The model under review builds one solid part; all positions refer to its coordinate system, in mm. Face numbers are marked on the shaded views. A direction names the side the tool comes from. Give positions to 0.01 mm unless a question says otherwise; leave off trailing zeros. Loops run counter-clockwise (first coordinate to the right, second up) from the corner with the lowest first, then second, coordinate; pieces in that order, holes last. Notation, with made-up numbers: (-12, -10) - (4, -10) arc R19 ccw to (4, 10) - close; hole circle Ø10 at (-25.75, -30.75). An arc over 180 degrees is marked (long way). Answer as a JSON object with one key per item and string values.
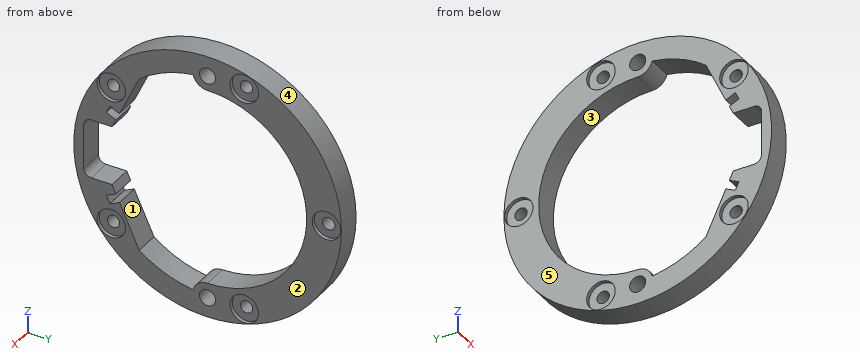
Autodesk Inventor part; units mm, degrees
ref_plane "YZ Plane" through (0, 0, 0) normal (1, 0, 0) x (0, 1, 0)
ref_plane "XZ Plane" through (0, 0, 0) normal (0, 1, 0) x (-1, 0, 0)
ref_plane "XY Plane" through (0, 0, 0) normal (0, 0, 1) x (1, 0, 0)
sketch "Sketch1" plane through (0, 0, 0) normal (1, 0, 0) x (0, 1, 0)
  circle A0 centre (-0.0138, -0.0327) radius 54
  circle A1 centre (-0.0138, 45.9673) radius 3.25
  circle A2 centre (-0.0138, -46.0327) radius 3.25
  arc A3 (-5.855, 44.5961) -> (-0.0138, 39.9673) centre (-0.0138, 45.9673) ccw
  arc A4 (-0.0138, -40.0327) -> (-5.8512, -44.6455) centre (-0.0138, -46.0327) ccw
  arc A5 (-0.0138, -40.0327) -> (-0.0138, 39.9673) centre (-0.0138, -0.0327) ccw
  line L0 (-38.5532, 11.9673) -> (-49.9975, 11.9673)
  line L1 (-49.9975, 11.9673) -> (-49.9975, -12.0327)
  line L2 (-38.5532, -12.0327) -> (-49.9975, -12.0327)
  arc A6 (-5.855, 44.5961) -> (-27.5449, 35.5747) centre (-0.0138, -0.0327) ccw
  arc A7 (-27.56, -35.6078) -> (-5.8512, -44.6455) centre (-0.0138, -0.0327) ccw
  line L3 (-36.9846, 15.3313) -> (-40.8817, 17.1485)
  line L4 (-40.8817, 17.1485) -> (-39.4448, 20.23)
  line L5 (-39.4448, 20.23) -> (-35.5477, 18.4127)
  line L6 (-35.5477, 18.4127) -> (-27.5449, 35.5747)
  line L7 (-36.9846, 15.3313) -> (-38.5532, 11.9673)
  line L8 (-36.9846, -15.3967) -> (-40.8817, -17.214)
  line L9 (-40.8817, -17.214) -> (-39.4448, -20.2954)
  line L10 (-39.4448, -20.2954) -> (-35.5477, -18.4782)
  line L11 (-36.9846, -15.3967) -> (-38.5532, -12.0327)
  line L12 (-35.5477, -18.4782) -> (-27.56, -35.6078)
  line L13 (-0.0138, -0.0327) -> (-40.1632, 18.6893)
  line L14 (-0.0138, -0.0327) -> (-40.1632, -18.7547)
  line L15 (-0.0138, -0.0327) -> (-50.798, -0.0327) construction
  line L16 (-0.0138, -0.0327) -> (50.7703, -0.0327) construction
  dimension "d4" = 6.5
  dimension "d5" = 6.5
  dimension "d25" = 24
  dimension "d27" = 4.3
  dimension "d28" = 3.4
  dimension "d31" = 4.3
  dimension "d32" = 3.4
  dimension "d39" = 90
  dimension "d40" = 90
  dimension "d41" = 90
  dimension "d42" = 90
  dimension "d44" = 90
  dimension "d45" = 90
  dimension "d67" = 40
  dimension "d68" = 40
  dimension "d70" = 4.3
  dimension "d71" = 1.7
  dimension "d72" = 4.3
  dimension "d73" = 90
  dimension "d74" = 90
  dimension "d76" = 108
  dimension "d81" = 40
  dimension "d93" = 46
  dimension "d94" = 46
  dimension "d95" = 6
  dimension "d96" = 6
  dimension "d97" = 180
  dimension "d98" = 12
  dimension "d99" = 12
  dimension "d100" = 25
  dimension "d101" = 25
  dimension "d102" = 1.7
extrude "Extrusion1" add sketch "Sketch1" along normal blind 10
fillet "Fillet1" radius 3 2 edges at (5, -49.9975, 11.9673) (5, -49.9975, -12.0327)
sketch "Sketch2" plane through (10, -0.0138, -0.0327) normal (1, 0, 0) x (0, 0, -1)
  circle A0 centre (0, 0) radius 48
  circle A1 centre (0, 48) radius 2.5
  arc A2 (40, 0) -> (-40, 0) centre (0, 0) ccw
  arc A3 (40, 0) -> (44.6128, -5.8374) centre (46, 0) ccw
  arc A4 (35.575, -27.5462) -> (44.6128, -5.8374) centre (0, 0) ccw
  line L0 (35.575, -27.5462) -> (18.4455, -35.5339)
  line L1 (18.4455, -35.5339) -> (20.2627, -39.431)
  line L2 (20.2627, -39.431) -> (17.1813, -40.8679)
  line L3 (17.1813, -40.8679) -> (15.364, -36.9708)
  line L4 (15.364, -36.9708) -> (12, -38.5394)
  line L5 (12, -38.5394) -> (12, -46.9837)
  arc A5 (9, -49.9837) -> (12, -46.9837) centre (9, -46.9837) ccw
  line L6 (9, -49.9837) -> (-9, -49.9837)
  arc A6 (-12, -46.9837) -> (-9, -49.9837) centre (-9, -46.9837) ccw
  line L7 (-12, -46.9837) -> (-12, -38.5394)
  line L8 (-12, -38.5394) -> (-15.364, -36.9708)
  line L9 (-15.364, -36.9708) -> (-17.1813, -40.8679)
  line L10 (-17.1813, -40.8679) -> (-20.2627, -39.431)
  line L11 (-20.2627, -39.431) -> (-18.4455, -35.5339)
  line L12 (-18.4455, -35.5339) -> (-35.6074, -27.5311)
  arc A7 (-44.6288, -5.8412) -> (-35.6074, -27.5311) centre (0, 0) ccw
  arc A8 (-44.6288, -5.8412) -> (-40, 0) centre (-46, 0) ccw
  circle A9 centre (46, 0) radius 3.25
  circle A10 centre (-46, 0) radius 3.25
  circle A11 centre (0, 0) radius 54
  circle A12 centre (0, 0) radius 54
  circle A13 centre (-45.6507, 14.8328) radius 2.5
  circle A14 centre (-28.2137, -38.8328) radius 2.5
  circle A15 centre (28.2137, -38.8328) radius 2.5
  circle A16 centre (45.6507, 14.8328) radius 2.5
  point P0 (-0.0327, 0.0138)
  dimension "d50" = 96
  dimension "d51" = 5
  dimension "d80" = 108
  dimension "d84" = 360
  dimension "d103" = 0
extrude "Extrusion2" cut sketch "Sketch2" against normal blind 10 contours A16 A0 | A0 A16 | A15 A0 | A0 A15 | A1 A0 | A0 A1 | A13 A0 | A0 A13 | A14 A0 | A0 A14
sketch "Sketch3" plane through (10, -0.0138, -0.0327) normal (1, 0, 0) x (0, 0, -1)
  circle A0 centre (0, 48) radius 2.5
  circle A1 centre (0, 48) radius 5.75
  circle A2 centre (0, 0) radius 54
  circle A3 centre (-45.6507, 14.8328) radius 5.75
  circle A4 centre (-28.2137, -38.8328) radius 5.75
  circle A5 centre (28.2137, -38.8328) radius 5.75
  circle A6 centre (45.6507, 14.8328) radius 5.75
  point P0 (-0.0327, 0.0138)
  dimension "d58" = 11.5
  dimension "d88" = 360
extrude "Extrusion3" cut sketch "Sketch3" against normal blind 1.5 contours A1 | A3 | A4 | A5 | A6
sketch "Sketch6" plane through (0, -0.0138, -0.0327) normal (-1, 0, 0) x (0, 0, 1)
  circle A0 centre (0, 48) radius 5.75
  circle A1 centre (-45.6507, 14.8328) radius 5.75
  circle A2 centre (-28.2137, -38.8328) radius 5.75
  circle A3 centre (28.2137, -38.8328) radius 5.75
  circle A4 centre (45.6507, 14.8328) radius 5.75
  point P0 (0.0327, 0.0138)
extrude "Extrusion5" cut sketch "Sketch6" against normal blind 1.5
equation "\"d98\" = 0.5 * d25"
properties part number "3219_Center Rung_V1" material "Acetal Resin, White"
Q1. Consider section A-A, the plane z = 29. State the section outline as (x, y) points, plus the area to 3 significant figures.
Results:
{"outline": "(0, -45.55) - (10, -45.55) - (10, -44.54) - (8.5, -44.54) - (8.5, -41.21) - (1.5, -41.21) - (1.5, -44.54) - (0, -44.54) - close; (0, -33.16) - (1.5, -33.16) - (1.5, -36.48) - (8.5, -36.48) - (8.5, -33.16) - (10, -33.16) - (10, -30.61) - (0, -30.61) - close; (0, 27.5) - (10, 27.5) - (10, 45.52) - (0, 45.52) - close", "area": "262 mm^2"}
Q2. Clearance check with flat-ended pins moving along their axes: pin 1 Ø6 at (y, z) = (13, -44) entering from +X; pin 2 Ø5 at (x, z) = (5.5, 33) entering from +Y; pin 3 Ø5 at (x, y) = (3, -9) entering from +Z. State where each tip first meets the part, or that it passes through.
Results:
{"pin 1": "stops at x = 8.5", "pin 2": "stops at y = 44.53", "pin 3": "stops at z = 53.58"}
Q3. Consider section C-C, the plane x = 5. State how many separate pieces and enclosed holes the cut face has, plus the area to 3 significant figures.
Results:
{"separate pieces": "1", "enclosed holes": "8", "area": "3,390 mm^2"}
Q4. For the marked faces 1 and 2, list the 3-axis set-ups (+Z, -Z, +X, -X, +Y, -Y) from which the entire face can be reached by the end or side of a thin tool; tool diameter is ignored.
Results:
{"face 1": "+X, -X", "face 2": "+Z, -Z, +X, +Y, -Y"}
Q5. The part is to be moulded in two halves that separate along Z. For the marked faces 3, 4 and 5, say which applies: +Z half, -Z half, draft (parallel to the pull), parting line (faces both ways), or undercut.
Results:
{"face 3": "undercut", "face 4": "parting line", "face 5": "draft"}
Q6. To check wall thickness, follow probe 1 along Y at (x, z) = (8.25, 1); probe 2 along Y at (x, z) = (3.75, 29); probe 3 along Z at (x, y) = (9, -12). State the ranges of each line that lie inside material, in increasing order. Write a range as [from, to].
Results:
{"probe 1": "y = [-54, -50], [39.97, 45.71], [50.26, 53.98]", "probe 2": "y = [-45.55, -41.21], [-36.48, -30.61], [27.5, 45.52]", "probe 3": "z = [-52.69, -43.4], [43.35, 52.62]"}
Q7. Consider section B-B, the plane y = 35.5. State the section outline as (x, z) points.
Results:
{"outline": "(0, -40.71) - (10, -40.71) - (10, -18.44) - (0, -18.44) - close; (0, 18.37) - (10, 18.37) - (10, 40.65) - (0, 40.65) - close"}
Q8. Consider section D-D, the plane y = -14.5. State the section outline as (x, z) points, plus the area to 3 significant figures.
Results:
{"outline": "(0, -52.05) - (10, -52.05) - (10, -42.63) - (0, -42.63) - close; (0, 42.58) - (10, 42.58) - (10, 51.99) - (0, 51.99) - close", "area": "188 mm^2"}
